```python
from build123d import *

# Parameters (mm, degrees)
SKETCH2_R                = 33.8
CUT_EXTRUDE1_DEPTH       = 19.1
CUT_EXTRUDE2_START       = -33.8
CUT_EXTRUDE2_DEPTH       = 14.7
BOSS_EXTRUDE2_START      = -1.7
BOSS_EXTRUDE2_DEPTH      = 1.7
SKETCH19_R               = 9
CUT_EXTRUDE10_DEPTH      = 1.4
CUT_EXTRUDE11_REACH      = 42.429
CUT_EXTRUDE11_END_RADIUS = 33.8
SKETCH20_R               = 3.5
CUT_EXTRUDE7_REACH       = 44.024
CUT_EXTRUDE7_END_RADIUS  = 33.8
SKETCH10_R               = 1.6
CUT_EXTRUDE12_REACH      = 42.714
SKETCH21_R               = 27.886018002


# Read off the part's stored shape, not the designer's step: Revolve2
with BuildPart() as part:
    # Sketch1 → Revolve1 (revolve)
    with BuildSketch(Plane.XY, mode=Mode.PRIVATE) as revolve1_sk:
        with BuildLine():
            Line((0, -33.8), (0, 0))
            Line((0, 0), (33.8, 0))
            ThreePointArc((33.8, 0), (23.900209204, -23.900209204), (0, -33.8))
        make_face()
    revolve(revolve1_sk.sketch.rotate(Axis((0, -33.8, 0), (0, 1, 0)), 180), axis=Axis((0, -33.8, 0), (0, 1, 0)))

    # Sketch2 → Cut-Extrude1 (cut)
    with BuildSketch(Plane(origin=(0, 0, 0), x_dir=(1, 0, 0), z_dir=(0, 1, 0))):
        Circle(SKETCH2_R)
    extrude(amount=-CUT_EXTRUDE1_DEPTH, mode=Mode.SUBTRACT)

    # Sketch5 → Cut-Extrude2 (cut)
    with BuildSketch(Plane(origin=(0, 0, 0), x_dir=(1, 0, 0), z_dir=(0, 1, 0)).offset(CUT_EXTRUDE2_START)):
        with BuildLine():
            Line((-17.025732229, 6.571677263), (-23.544283672, 3.742739979))
            ThreePointArc((-23.544283672, 3.742739979), (-23.775794442, 3.633514413), (-24, 3.509985755))
            Line((-24, 3.509985755), (-24, -3.509985755))
            ThreePointArc((-24, -3.509985755), (-23.775794442, -3.633514413), (-23.544283672, -3.742739979))
            Line((-23.544283672, -3.742739979), (-17.025732229, -6.571677263))
            ThreePointArc((-17.025732229, -6.571677263), (0, -18.25), (17.025732229, -6.571677263))
            Line((17.025732229, -6.571677263), (23.544283672, -3.742739979))
            ThreePointArc((23.544283672, -3.742739979), (23.775794442, -3.633514413), (24, -3.509985755))
            Line((24, -3.509985755), (24, 3.509985755))
            ThreePointArc((24, 3.509985755), (23.775794442, 3.633514413), (23.544283672, 3.742739979))
            Line((23.544283672, 3.742739979), (17.025732229, 6.571677263))
            ThreePointArc((17.025732229, 6.571677263), (0, 18.25), (-17.025732229, 6.571677263))
        make_face()
    extrude(amount=CUT_EXTRUDE2_DEPTH, mode=Mode.SUBTRACT)

    # Sketch16 → Boss-Extrude2 (add)
    with BuildSketch(Plane(origin=(0, -19.1, 0), x_dir=(1, 0, 0), z_dir=(0, 1, 0)).offset(BOSS_EXTRUDE2_START)):
        with BuildLine():
            Line((17.025732229, 6.571677263), (23.544283672, 3.742739979))
            ThreePointArc((23.544283672, 3.742739979), (23.775794442, 3.633514413), (24, 3.509985755))
            Line((24, 3.509985755), (24, -3.509985755))
            ThreePointArc((24, -3.509985755), (23.775794442, -3.633514413), (23.544283672, -3.742739979))
            Line((23.544283672, -3.742739979), (17.025732229, -6.571677263))
            ThreePointArc((17.025732229, -6.571677263), (18.25, 0), (17.025732229, 6.571677263))
        make_face()
        with BuildLine():
            Line((-23.544283672, -3.742739979), (-17.025732229, -6.571677263))
            ThreePointArc((-17.025732229, -6.571677263), (-18.25, 0), (-17.025732229, 6.571677263))
            Line((-17.025732229, 6.571677263), (-23.544283672, 3.742739979))
            ThreePointArc((-23.544283672, 3.742739979), (-23.775794442, 3.633514413), (-24, 3.509985755))
            Line((-24, 3.509985755), (-24, -3.509985755))
            ThreePointArc((-24, -3.509985755), (-23.775794442, -3.633514413), (-23.544283672, -3.742739979))
        make_face()
    extrude(amount=BOSS_EXTRUDE2_DEPTH)

    # Revolve2 outline → Revolve2 (revolve)
    with BuildSketch(Plane.XY):
        with BuildLine():
            Line((0, -23.5), (0, -33.8))
            ThreePointArc((0, -33.8), (13.168073663, -31.129436808), (24.255308697, -23.53975361))
            Line((24.255308697, -23.53975361), (24.255308697, -23.5))
            Line((24.255308697, -23.5), (0, -23.5))
        make_face()
    revolve(axis=Axis((0, 0, 0), (0, 1, 0)))

    # Sketch19 → Cut-Extrude10 (cut)
    with BuildSketch(Plane(origin=(0, -23.5, 0), x_dir=(1, 0, 0), z_dir=(0, 1, 0))):
        with Locations(Location((0, 0, 0), (0, 0, 180))):
            Circle(SKETCH19_R)
    extrude(amount=-CUT_EXTRUDE10_DEPTH, mode=Mode.SUBTRACT)

    # Cut-Extrude11: up to this sphere (the profile starts inside it)
    cut_extrude11_end = Location((0, 0, 0)) * Sphere(CUT_EXTRUDE11_END_RADIUS, mode=Mode.PRIVATE)
    # Sketch20 → Cut-Extrude11 (cut, up to the surface)
    with BuildSketch(Plane(origin=(0, -24.9, 0), x_dir=(1, 0, 0), z_dir=(0, 1, 0)), mode=Mode.PRIVATE) as cut_extrude11_sk1:
        with Locations(Location((0, 0, 0), (0, 0, 180))):
            Circle(SKETCH20_R)
    cut_extrude11_tool1 = extrude(cut_extrude11_sk1.sketch, amount=-CUT_EXTRUDE11_REACH, mode=Mode.PRIVATE) & cut_extrude11_end
    add(cut_extrude11_tool1.solids().sort_by_distance((0, -24.9, 0))[0], mode=Mode.SUBTRACT)

    # Cut-Extrude7: up to this sphere (the profile starts inside it)
    cut_extrude7_end = Location((0, 0, 0)) * Sphere(CUT_EXTRUDE7_END_RADIUS, mode=Mode.PRIVATE)
    # Sketch10 → Cut-Extrude7 (cut, up to the surface)
    with BuildSketch(Plane(origin=(0, -19.1, 0), x_dir=(1, 0, 0), z_dir=(0, 1, 0)), mode=Mode.PRIVATE) as cut_extrude7_sk1:
        with Locations(Location((-18.186533479, -10.5, 0), (0, 0, 270))):
            Circle(SKETCH10_R)
    cut_extrude7_tool1 = extrude(cut_extrude7_sk1.sketch, amount=-CUT_EXTRUDE7_REACH, mode=Mode.PRIVATE) & cut_extrude7_end
    add(cut_extrude7_tool1.solids().sort_by_distance((-18.186533, -19.1, 10.5))[0], mode=Mode.SUBTRACT)
    # Sketch10 → Cut-Extrude7 (cut, up to the surface)
    with BuildSketch(Plane(origin=(0, -19.1, 0), x_dir=(1, 0, 0), z_dir=(0, 1, 0)), mode=Mode.PRIVATE) as cut_extrude7_sk2:
        with Locations(Location((18.186533479, 10.5, 0), (0, 0, 270))):
            Circle(SKETCH10_R)
    cut_extrude7_tool2 = extrude(cut_extrude7_sk2.sketch, amount=-CUT_EXTRUDE7_REACH, mode=Mode.PRIVATE) & cut_extrude7_end
    add(cut_extrude7_tool2.solids().sort_by_distance((18.186533, -19.1, -10.5))[0], mode=Mode.SUBTRACT)

    # Sketch21 → Cut-Extrude12 (cut, up to next)
    with BuildSketch(Plane(origin=(0, -23.5, 0), x_dir=(1, 0, 0), z_dir=(0, 1, 0)), mode=Mode.PRIVATE) as cut_extrude12_sk1:
        Circle(SKETCH21_R)
    cut_extrude12_tool1 = extrude(cut_extrude12_sk1.sketch, amount=CUT_EXTRUDE12_REACH, mode=Mode.PRIVATE) & part.part
    add(cut_extrude12_tool1.solids().sort_by_distance((0, -23.5, 0))[0], mode=Mode.SUBTRACT)


solid = part.part
```
The model under review builds one solid part; all positions refer to its coordinate system, in mm. A direction names the side the tool comes from. Round coordinates to 2 decimals unless told otherwise and drop trailing zeros. Loops run counter-clockwise (first coordinate to the right, second up) from the corner with the lowest first, then second, coordinate; pieces in that order, holes last.
Item 1: Take a section at D-D (z = 10.5). Write out the cut boundary in (x, y).
Determined:
outline: (-21.91, -23.5) arc R32.13 ccw to (-19.79, -25.31) - (-19.79, -23.5) - close; (-16.59, -27.52) arc R32.13 ccw to (21.91, -23.5) - (-16.59, -23.5) - close
Item 2: Take a section at B-B (z = 0). Write out the cut boundary in (x, y), then the cut area to 3 significant figures.
Determined:
outline: (-24.29, -23.5) arc R33.8 ccw to (-3.5, -33.62) - (-3.5, -24.9) - (-9, -24.9) - (-9, -23.5) - close; (3.5, -33.62) arc R33.8 ccw to (24.29, -23.5) - (9, -23.5) - (9, -24.9) - (3.5, -24.9) - close
area: 258 mm2
Item 3: Clearance check with flat-ended pins moving along their axes: pin 1 Ø2 at (x, y) = (5, -28) entering from -Z; pin 2 Ø3 at (y, z) = (-27.5, -7.5) entering from +X; pin 3 Ø3 at (x, y) = (6.5, -31.5) entering from +Z. State where each tip first meets the part, or that it passes through.
Determined:
pin 1: stops at z = -19.73
pin 2: stops at x = 20.33
pin 3: stops at z = 14.22
Item 4: For faces 1 (the face through (-16.6, -25.1, 10.3)), 2 (the face through (0, -24.9, -4)), list the 3-axis set-ups (+Z, -Z, +X, -X, +Y, -Y) from which the entire face can be reached by the end or side of a thin tool; tool diameter is ignored.
Determined:
face 1: +Y, -Y
face 2: +Y
Item 5: For line 1 (Z direction, x = 0, y = -24.3); line 2 (X direction, y = -24.35, z = -10.5); line 3 (X direction, y = -26.75, z = 0.5), list the stretches that pass through material, from the lowest coordinate up.
Determined:
line 1: z = -23.49 to -9, 9 to 23.49
line 2: x = -20.96 to 16.59, 19.79 to 20.96
line 3: x = -20.65 to -3.46, 3.46 to 20.65
Item 6: Take a section at C-C (y = -31.25). Write out the cut boundary in (x, z).
Determined:
outline: circle Ø25.76 at (0, 0); hole circle Ø7 at (0, 0)
Item 7: Take a section at A-A (x = 0). Write out the cut boundary in (y, z), then the cut area to 3 significant figures.
Determined:
outline: (-33.62, -3.5) arc R33.8 ccw to (-23.5, -24.29) - (-23.5, -9) - (-24.9, -9) - (-24.9, -3.5) - close; (-33.62, 3.5) - (-24.9, 3.5) - (-24.9, 9) - (-23.5, 9) - (-23.5, 24.29) arc R33.8 ccw to start
area: 258 mm2
Item 8: Mouldability with a two-part tool opening along Z and no side actions: class faces 3 (the face through (16.77, -25.1, -9.76)), 4 (the face through (10, -23.5, 0)) as released by +Z, released by -Z, zero draft, split by the parting line, or undercut.
Determined:
face 3: undercut
face 4: zero draft
